Verification items for the finished model (mm, model axes). Face numbers are marked on the shaded views. A direction names the side the tool comes from. Give positions to 0.01 mm unless a question says otherwise; leave off trailing zeros. Write each loop counter-clockwise with the first axis right and the second up, starting at its lowest first coordinate (ties: lowest second). Pieces come first, ordered by that corner, then holes. Notation, with made-up numbers: (48, 39.25) - (68, 39.25) arc R9 cw to (68, 49.25) - close; hole circle Ø9 at (38.25, 79). An arc over 180 degrees is marked (long way). Put each result on its own line as item: value.
from build123d import *

# Parameters (mm, degrees)
BOSS_EXTRUDE1_DEPTH  = 8
BOSS_EXTRUDE3_DEPTH  = 109
M3_CLEARANCE_SLOT1_D = 3.2


with BuildPart() as part:
    # Sketch1 → Boss-Extrude1 (new body)
    with BuildSketch(Plane.XY):
        with BuildLine():
            Line((15, 25.5), (-15, 25.5))
            Line((-15, 25.5), (-15, -7))
            Line((-15, -7), (-5, -15.660254038))
            ThreePointArc((-5, -15.660254038), (0, -17), (5, -15.660254038))
            Line((5, -15.660254038), (15, -7))
            Line((15, -7), (15, 25.5))
        make_face()
        with BuildLine():
            Line((1.658312395, -4.5), (-1.658312395, -4.5))
            ThreePointArc((-1.658312395, -4.5), (0, -10), (1.658312395, -4.5))
        make_face(mode=Mode.SUBTRACT)
    extrude(amount=BOSS_EXTRUDE1_DEPTH)

    # Sketch1<5> → Boss-Extrude3 (add)
    with BuildSketch(Plane.XY):
        Polygon((-12.5, 28), (12.5, 28), (15, 25.5), (-15, 25.5), align=None)
    extrude(amount=BOSS_EXTRUDE3_DEPTH)

    # M3 Clearance Slot1 (through all)
    with Locations(Plane(origin=(0, 28, 0), x_dir=(1, 0, 0), z_dir=(0, 1, 0))):
        with Locations((-8.5, -15), (8.5, -15), (-8.5, -102), (8.5, -102)):
            Hole(M3_CLEARANCE_SLOT1_D / 2)


solid = part.part
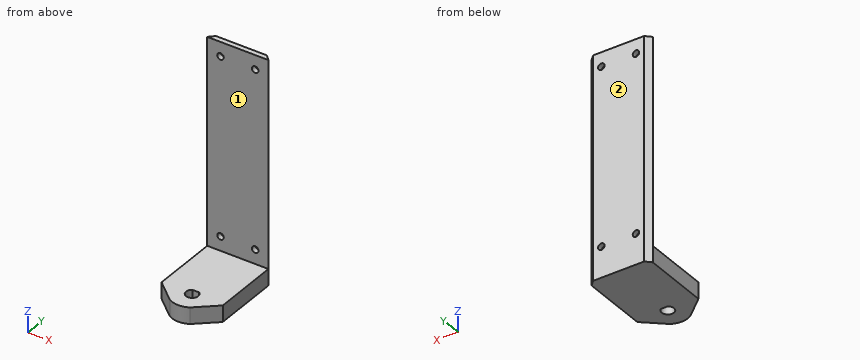
Q1. Section check A-A, the plane x = 0. Record the cut outline in (y, z).
Answers follow:
outline: (-17, 0) - (-10, 0) - (-10, 8) - (-17, 8) - close; (-4.5, 0) - (28, 0) - (28, 109) - (25.5, 109) - (25.5, 8) - (-4.5, 8) - close
Q2. Section check C-C, the plane x = 8.5. Record the cut outline in (y, z).
Answers follow:
outline: (-12.63, 0) - (28, 0) - (28, 13.4) - (25.5, 13.4) - (25.5, 8) - (-12.63, 8) - close; (25.5, 16.6) - (28, 16.6) - (28, 100.4) - (25.5, 100.4) - close; (25.5, 103.6) - (28, 103.6) - (28, 109) - (25.5, 109) - close
Q3. Go/stop test with flat-tipped pins: pin 1 Ø6 at (x, y) = (10.5, -6.5) entering from +Z; pin 2 Ø2.5 at (x, z) = (-8.5, 15) entering from -Y; pin 3 Ø5 at (x, z) = (8.5, 102) entering from -Y. Record where each tip stops, or that it passes through.
Answers follow:
pin 1: stops at z = 8
pin 2: passes through
pin 3: stops at y = 25.5
Q4. Set-up check for the marked faces 1 and 2: record each of +Z, -Z, +X, -X, +Y, -Y from which the full face is reachable in a straight line by a thin tool's end or side.
Answers follow:
face 1: +Z, +X, -X, -Y
face 2: +Z, -Z, +X, -X, +Y
Q5. Section check D-D, the plane z = 36. Record the cut outline in (x, y), plus the area to 4 significant figures.
Answers follow:
outline: (-15, 25.5) - (15, 25.5) - (12.5, 28) - (-12.5, 28) - close
area: 68.75 mm2
Q6. Section check B-B, the plane z = 15. Record the cut outline in (x, y), plus the area to 4 significant figures.
Answers follow:
outline: (-15, 25.5) - (-10.1, 25.5) - (-10.1, 28) - (-12.5, 28) - close; (-6.9, 25.5) - (6.9, 25.5) - (6.9, 28) - (-6.9, 28) - close; (10.1, 25.5) - (15, 25.5) - (12.5, 28) - (10.1, 28) - close
area: 52.75 mm2
Q7. Scan lines: line 1 along Z through (x, y) = (-8.5, 26.25); line 2 along X through (y, z) = (-7, 2); line 3 along X through (y, z) = (26.35, 102). Record each from-to range of solid material in increasing order.
Answers follow:
line 1: z = 0 to 13.4, 16.6 to 100.4, 103.6 to 109
line 2: x = -15 to -3, 3 to 15
line 3: x = -14.15 to -10.1, -6.9 to 6.9, 10.1 to 14.15
